Verification items for the finished model (mm, model axes). Face numbers are marked on the shaded views. A direction names the side the tool comes from. Give positions to 0.01 mm unless a question says otherwise; leave off trailing zeros. Loops run counter-clockwise (first coordinate to the right, second up) from the corner with the lowest first, then second, coordinate; pieces in that order, holes last. Notation, with made-up numbers: (62.5, -7) -> (79.5, -7) arc R11 ccw to (79.5, 4) -> close; hole circle Ø3 at (-1.5, 36). An arc over 180 degrees is marked (long way). Answer in a Markdown table with one row per item. Add a question column.
Q1. Set-up check for the marked faces 1, 2 and 3: record each of +Z, -Z, +X, -X, +Y, -Y from which the full face is reachable in a straight line by a thin tool's end or side.
Q2. Section check C-C on x = 6. Enter the section's corners in (y, z), and give its area (3 significant figures).
Q3. Section check B-B on y = 20. Enter the section's corners in (x, z).
Q4. Section check A-A on z = 22. Enter the section's corners in (x, y), and give its area (3 significant figures).
Q5. Gauge pin test, flat ends, axial feed: P1, Ø8, axis at x = 4, y = 45.5, coming from the +Z side; P2, Ø2.5, axis at x = 8, z = 24, coming from the +Y side; P3, Ø3, axis at y = 38.5, z = -17, coming from the -X side. Record the tip position at first contact, or that the pin passes through.
Q6. Material ranges on probe 1 along X at (y, z) = (-1, 0); probe 2 along Z at (x, y) = (-0.5, 23); probe 3 along Y at (x, z) = (-10.5, 20), recorded low to high.
```python
from build123d import *

# Parameters (mm, degrees)
IZIM1_R                     = 27.5
Y_KSEKLIK_EKSTR_ZYON1_DEPTH = 2
IZIM2_R                     = 25
IZIM2_R_2                   = 23
Y_KSEKLIK_EKSTR_ZYON2_DEPTH = 3
Y_KSEKLIK_EKSTR_ZYON3_DEPTH = 50.8
PAH1_SIZE                   = 8
PAH1_SIZE_2                 = 21.979819356
PAH2_SIZE                   = 8
PAH2_SIZE_2                 = 21.979819356
IZIM4_R                     = 3.5
Y_KSEKLIK_EKSTR_ZYON4_DEPTH = 4
Y_KSEKLIK_EKSTR_ZYON5_START = 4
IZIM5_R                     = 3.5
Y_KSEKLIK_EKSTR_ZYON5_DEPTH = 4


with BuildPart() as part:
    # Çizim1 → Yükseklik-Ekstrüzyon1 (new body)
    with BuildSketch(Plane(origin=(0, 0, 0), x_dir=(1, 0, 0), z_dir=(0, 1, 0))):
        with Locations(Location((0, 0, 0), (0, 0, 270))):
            Circle(IZIM1_R)
    extrude(amount=Y_KSEKLIK_EKSTR_ZYON1_DEPTH)

    # Çizim2 → Yükseklik-Ekstrüzyon2 (add)
    with BuildSketch(Plane.XZ):
        with Locations(Location((0, 0, 0), (0, 0, 90))):
            Circle(IZIM2_R)
        with Locations(Location((0, 0, 0), (0, 0, 270))):
            Circle(IZIM2_R_2, mode=Mode.SUBTRACT)
    extrude(amount=Y_KSEKLIK_EKSTR_ZYON2_DEPTH)

    # Çizim3 → Yükseklik-Ekstrüzyon3 (add)
    with BuildSketch(Plane(origin=(0, 2, 0), x_dir=(1, 0, 0), z_dir=(0, 1, 0))):
        with BuildLine():
            Line((-17.5, -19), (17.5, -19))
            ThreePointArc((17.5, -19), (24.571067812, -16.071067812), (27.5, -9))
            Line((27.5, -9), (27.5, 9))
            ThreePointArc((27.5, 9), (24.571067812, 16.071067812), (17.5, 19))
            Line((17.5, 19), (-17.5, 19))
            ThreePointArc((-17.5, 19), (-24.571067812, 16.071067812), (-27.5, 9))
            Line((-27.5, 9), (-27.5, -9))
            ThreePointArc((-27.5, -9), (-24.571067812, -16.071067812), (-17.5, -19))
        make_face()
    extrude(amount=Y_KSEKLIK_EKSTR_ZYON3_DEPTH)

    # Pah1
    # the kernel refuses this chamfer: 21.979819356, 8 mm, written as the material it takes off along each edge
    with BuildSketch(Plane(origin=(74.519931595, 52.8, -19), x_dir=(0, -0.9950833631817486, -0.0990409022520504), z_dir=(-1, 0, 0))) as pah1_piece_1:
        Polygon((PAH1_SIZE * 0.995083363182, PAH1_SIZE * 0.0990409022521), (-PAH1_SIZE_2 * 0.0990409022504, PAH1_SIZE_2 * 0.995083363165), (0, 0), align=None)
    extrude(amount=149.03986319, mode=Mode.SUBTRACT)

    # Pah2
    # the kernel refuses this chamfer: 21.979819356, 8 mm, written as the material it takes off along each edge
    with BuildSketch(Plane(origin=(-74.519931595, 52.8, 19), x_dir=(0, -0.9950833631817486, 0.0990409022520504), z_dir=(1, 0, 0))) as pah2_piece_1:
        Polygon((PAH2_SIZE * 0.995083363182, PAH2_SIZE * 0.0990409022521), (-PAH2_SIZE_2 * 0.0990409022504, PAH2_SIZE_2 * 0.995083363165), (0, 0), align=None)
    extrude(amount=149.03986319, mode=Mode.SUBTRACT)

    # Çizim4 → Yükseklik-Ekstrüzyon4 (add)
    with BuildSketch(Plane.XY.offset(19)):
        with Locations(Location((0, 38, 0), (0, 0, 180))):
            Circle(IZIM4_R)
    extrude(amount=Y_KSEKLIK_EKSTR_ZYON4_DEPTH)

    # Çizim5 → Yükseklik-Ekstrüzyon5 (add)
    with BuildSketch(Plane(origin=(0, 0, -19), x_dir=(-1, 0, 0), z_dir=(0, 0, -1)).offset(Y_KSEKLIK_EKSTR_ZYON5_START)):
        with Locations((0, 38)):
            Circle(IZIM5_R)
    extrude(amount=-Y_KSEKLIK_EKSTR_ZYON5_DEPTH)


solid = part.part
```
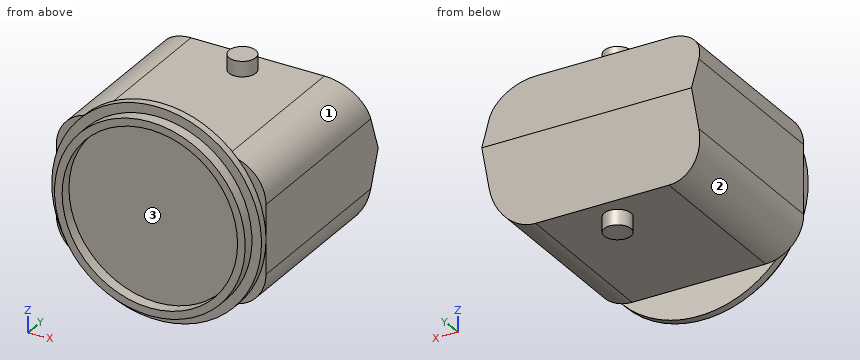
Taken from the geometry:
| question | item | result |
|---|---|---|
| 1 | face 1 | +Z, +X, +Y |
| 1 | face 2 | -Z, -X, +Y |
| 1 | face 3 | -Y |
| 2 | outline | (-3, -24.27) -> (0, -24.27) -> (0, -26.84) -> (2, -26.84) -> (2, -19) -> (44.8, -19) -> (51.72, 0) -> (44.8, 19) -> (2, 19) -> (2, 26.84) -> (0, 26.84) -> (0, 24.27) -> (-3, 24.27) -> (-3, 22.2) -> (0, 22.2) -> (0, -22.2) -> (-3, -22.2) -> close |
| 2 | area | 1,880 mm² |
| 3 | outline | (-27.5, -9) arc R10 ccw to (-17.5, -19) -> (17.5, -19) arc R10 ccw to (27.5, -9) -> (27.5, 9) arc R10 ccw to (17.5, 19) -> (-17.5, 19) arc R10 ccw to (-27.5, 9) -> close |
| 4 | outline | (-16.5, 0) -> (-11.87, 0) -> (-11.87, -3) -> (-6.71, -3) -> (-6.71, 0) -> (6.71, 0) -> (6.71, -3) -> (11.87, -3) -> (11.87, 0) -> (16.5, 0) -> (16.5, 2) -> (-16.5, 2) -> close; circle Ø7 at (0, 38) |
| 4 | area | 135 mm² |
| 5 | P1 | stops at z = 19 |
| 5 | P2 | stops at y = 2 |
| 5 | P3 | stops at x = -25.1 |
| 6 | probe 1 | x = -25 to -23, 23 to 25 |
| 6 | probe 2 | z = -19 to 19 |
| 6 | probe 3 | y = 0 to 2 |
